from build123d import *

# Parameters (mm, degrees)
RETAINING_SCREW_HOLES_DEPTH      = 113.83205248
RETAINING_SCREW_HOLES_DEPTH_BACK = 113.83205248
SKETCH3_R                        = 2.5


with BuildPart() as part:
    # Ceiling structural member cradle: sweep along a path in Sketch2
    with BuildLine(Plane(origin=(0, 0, 0), x_dir=(1, 0, 0), z_dir=(0, 1, 0))) as ceiling_structural_member_cradle_path:
        ThreePointArc((-100, -3), (0, 0), (100, -3))
    # Sketch1 → Ceiling structural member cradle (sweep)
    with BuildSketch(Plane(origin=(0, 0, 0), x_dir=(0, 0, -1), z_dir=(1, 0, 0))):
        with BuildLine():
            Line((0, 0), (-37, 0))
            ThreePointArc((-37, 0), (-39.121320344, 0.878679656), (-40, 3))
            Line((-40, 3), (-40, 9))
            ThreePointArc((-40, 9), (-40.292893219, 9.707106781), (-41, 10))
            Line((-41, 10), (-42, 10))
            ThreePointArc((-42, 10), (-42.707106781, 9.707106781), (-43, 9))
            Line((-43, 9), (-43, 3))
            ThreePointArc((-43, 3), (-41.242640687, -1.242640687), (-37, -3))
            Line((-37, -3), (37, -3))
            ThreePointArc((37, -3), (41.242640687, -1.242640687), (43, 3))
            Line((43, 3), (43, 9))
            ThreePointArc((43, 9), (42.707106781, 9.707106781), (42, 10))
            Line((42, 10), (41, 10))
            ThreePointArc((41, 10), (40.292893219, 9.707106781), (40, 9))
            Line((40, 9), (40, 3))
            ThreePointArc((40, 3), (39.121320344, 0.878679656), (37, 0))
            Line((37, 0), (0, 0))
        make_face()
    sweep(path=ceiling_structural_member_cradle_path.line)

    # Sketch3 → Retaining screw holes (cut, two sides: drawn at the far end of the back side and taken through both)
    with BuildSketch(Plane(origin=(0, 0, 0), x_dir=(1, 0, 0), z_dir=(0, 1, 0)).offset(-RETAINING_SCREW_HOLES_DEPTH_BACK)):
        with Locations(Location((-77, -1.778048193, 0), (0, 0, 270))):
            Circle(SKETCH3_R)
        with Locations(Location((77, -1.778048193, 0), (0, 0, 270))):
            Circle(SKETCH3_R)
    extrude(amount=RETAINING_SCREW_HOLES_DEPTH + RETAINING_SCREW_HOLES_DEPTH_BACK, mode=Mode.SUBTRACT)


solid = part.part
Design review of the part built by this model. Coordinates are the model's own, in mm. Coordinates: 2 decimals unless noted, no trailing zeros. Loops run counter-clockwise (first coordinate to the right, second up) from the corner with the lowest first, then second, coordinate; pieces in that order, holes last. Notation, with made-up numbers: (34, 36.25) - (43, 36.25) arc R15 cw to (43, 50.25) - close; hole circle Ø2 at (27.5, -24.75). An arc over 180 degrees is marked (long way). Use CSV: the item, a comma, the result in double quotes. Start each with the question number.
1. Mouldability with a two-part tool opening along X and no side actions: class faces 1 (the cylindrical face through (-1, 6, -40)), 2 (the cylindrical face through (-1, 6, 40)), 3 (the flat face through (-1, -3, 1)) as released by +X, released by -X, zero draft, split by the parting line, or undercut.
2. Add section B-B on z = 34. Give the boundary of the cut face in (x, y), plus the area to 3 significant figures.
3. Clearance check with flat-ended pins moving along their axes: pin 1 (2 mm diameter, centred on x = 40, z = -4, fed in from +Y); pin 2 (1.5 mm diameter, centred on x = 10, y = 3.5, fed in from +Z). State where each tip first meets the part, or that it passes through.
4. Add section C-C on z = -28.5. Give the boundary of the cut face in (x, y).
5. To check wall thickness, follow probe 1 along Y at (x, z) = (70, -21); probe 2 along Z at (x, y) = (18, 8.5); probe 3 along Z at (x, y) = (-81, 3). State the ranges of each line that lie inside material, in increasing order.
6. Add section A-A on y = 5.5. Give the boundary of the cut face in (x, z), plus the area to 3 significant figures.
Resolved:
1,face 1,"undercut"
1,face 2,"split by the parting line"
1,face 3,"zero draft"
2,outline,"(-98.14, -3) - (98.14, -3) - (98.14, 0) - (-98.14, 0) - close"
2,area,"589 mm2"
3,pin 1,"y = 0"
3,pin 2,"z = 43.04"
4,outline,"(-101.89, -3) - (101.89, -3) - (101.89, 0) - (-101.89, 0) - close"
5,probe 1,"-3 to 0"
5,probe 2,"-42.91 to -39.91, 40.1 to 43.1"
5,probe 3,"-41.08 to -38.08, 42.02 to 45.02"
6,outline,"(-102.58, -39.92) arc R1711.17 ccw to (102.58, -39.92) - (102.4, -36.93) arc R1708.17 cw to (-102.4, -36.93) - close; (-97.6, 42.93) arc R1628.17 ccw to (97.6, 42.93) - (97.42, 45.92) arc R1625.17 cw to (-97.42, 45.92) - close"
6,area,"1,200 mm2"
